from build123d import *

# Parameters (mm, degrees)
F0_W     = 95.043734
F0_H     = 101.66876
F1_DEPTH = 84.074
F2_R     = 27.594461
F3_T     = -2.54


with BuildPart() as f1:
    # F0 (on Top) → F1 (new body)
    with BuildSketch(Plane.XY):
        Rectangle(F0_W, F0_H)
    extrude(amount=F1_DEPTH)

    # F2
    f2_edges = [f1.edges().sort_by_distance(p)[0] for p in [
        (-47.521867, 0, 0),
    ]]
    fillet(f2_edges, radius=F2_R)

    # F3
    f3_openings = [f1.faces().sort_by_distance(p)[0] for p in [
        (0.863429, -50.83438, 42.785922),
        (0, 0, 84.074),
        (47.521867, 0, 42.037),
    ]]
    offset(amount=F3_T, openings=f3_openings)


solid = f1.part
For this review, take the finished solid that the model builds, in its own axes (mm). A direction names the side the tool comes from. Round coordinates to 2 decimals unless told otherwise and drop trailing zeros. Order: outer loops, then holes, each group sorted by start corner. A loop starts at its lowest first (then second) coordinate and runs counter-clockwise, first axis right, second up. Notation, with made-up numbers: (89.25, 9.25) -> (108.25, 9.25) arc R18 ccw to (108.25, 43.25) -> close; hole circle Ø5 at (-27, 27.25). An arc over 180 degrees is marked (long way). Write item = value, one per line. Start each with the question number.
1) Insertion check: pin 1 (5 mm diameter, centred on y = 5.5, z = 67.5, fed in from +X); pin 2 (1.5 mm diameter, centred on x = 38, y = 18, fed in from +Z); pin 3 (24.5 mm diameter, centred on x = -4.5, z = 61, fed in from -Y). Each pin has a flat end and moves straight along its axis. Give the tip position at first contact, or say it passes through.
2) Take a section at C-C on x = 7.5. State the section outline as (y, z) points.
3) Take a section at A-A on y = 32.5. State the section outline as (x, z) points, plus the area to 3 significant figures.
4) Tool access review of faces 4 (the face through (1, 48.294, 43)), 5 (the face through (-46, 23, 84.074)): name each direction out of +Z, -Z, +X, -X, +Y, -Y from which nothing blocks a thin tool from reaching the whole face with its end or side.
5) The part is to be moulded in two halves that separate along Y. For faces 1 (the face through (-1, 50.834, 41)), 2 (the face through (-35.4, -50.834, 7.6)), 3 (the face through (13, 1, 0)), say which applies: +Y half, -Y half, draft (parallel to the pull), parting line (faces both ways), or undercut.
6) To check wall thickness, follow line 1 (X direction, y = -13, z = 69); line 2 (Z direction, x = 41.5, y = 17); line 3 (Y direction, x = 27, z = 39.5). State the ranges of each line that lie inside material, in increasing order. Write a range as from..to.
7) Take a section at B-B on z = 76. State the section outline as (x, y) points, plus the area to 3 significant figures.
Verdict:
q1.pin_1 = -44.98
q1.pin_2 = 2.54
q1.pin_3 = 48.29
q2.outline = (-50.83, 0) -> (50.83, 0) -> (50.83, 84.07) -> (48.29, 84.07) -> (48.29, 2.54) -> (-50.83, 2.54) -> close
q3.outline = (-47.52, 27.59) arc R27.59 ccw to (-19.93, 0) -> (47.52, 0) -> (47.52, 2.54) -> (-19.93, 2.54) arc R25.05 cw to (-44.98, 27.59) -> (-44.98, 84.07) -> (-47.52, 84.07) -> close
q3.area = 420 mm2
q4.face_4 = +Z, +X, -Y
q4.face_5 = +Z, +X, -X, +Y, -Y
q5.face_1 = +Y half
q5.face_2 = -Y half
q5.face_3 = draft
q6.line_1 = -47.52..-44.98
q6.line_2 = 0..2.54
q6.line_3 = 48.29..50.83
q7.outline = (-47.52, -50.83) -> (-44.98, -50.83) -> (-44.98, 48.29) -> (47.52, 48.29) -> (47.52, 50.83) -> (-47.52, 50.83) -> close
q7.area = 493 mm2
